```python
from build123d import *

# Parameters (mm, degrees)
SKETCH1_W           = 24
SKETCH1_H           = 9
BOSS_EXTRUDE1_DEPTH = 75
FILLET1_R           = 1
FILLET2_R           = 3
SKETCH2_R           = 2.5
CUT_EXTRUDE1_DEPTH  = 6
SKETCH3_R           = 2.5
CUT_EXTRUDE2_DEPTH  = 10
SKETCH4_R           = 5
CUT_EXTRUDE3_DEPTH  = 4


with BuildPart() as part:
    # Sketch1 → Boss-Extrude1 (new body)
    with BuildSketch(Plane.XY):
        Polygon((-18, -4.5), (-12, -4.5), (-12, 4.5), (-12, 14.5), (-18, 14.5), align=None)
        Rectangle(SKETCH1_W, SKETCH1_H)
        Polygon((12, 4.5), (12, -4.5), (18, -4.5), (18, 24.5), (12, 24.5), align=None)
    extrude(amount=BOSS_EXTRUDE1_DEPTH)

    # Fillet1
    fillet1_edges = [part.edges().sort_by_distance(p)[0] for p in [
        (-12, 4.5, 37.5),
        (12, 4.5, 37.5),
    ]]
    fillet(fillet1_edges, radius=FILLET1_R)

    # Fillet2
    fillet2_edges = [part.edges().sort_by_distance(p)[0] for p in [
        (18, 10, 0),
        (-18, 5, 0),
        (18, 10, 75),
        (-18, 5, 75),
    ]]
    fillet(fillet2_edges, radius=FILLET2_R)

    # Sketch2 → Cut-Extrude1 (cut)
    with BuildSketch(Plane.ZY.offset(-12)):
        with Locations((37.5, 13.5)):
            Circle(SKETCH2_R)
    extrude(amount=-CUT_EXTRUDE1_DEPTH, mode=Mode.SUBTRACT)

    # Sketch3 → Cut-Extrude2 (cut)
    with BuildSketch(Plane(origin=(0, 4.5, 0), x_dir=(1, 0, 0), z_dir=(0, 1, 0))):
        with Locations(Location((0, -37.5, 0), (0, 0, 270))):
            Circle(SKETCH3_R)
        with Locations(Location((0, -7.5, 0), (0, 0, 270))):
            Circle(SKETCH3_R)
        with Locations(Location((0, -67.5, 0), (0, 0, 270))):
            Circle(SKETCH3_R)
    extrude(amount=-CUT_EXTRUDE2_DEPTH, mode=Mode.SUBTRACT)

    # Sketch4 → Cut-Extrude3 (cut)
    with BuildSketch(Plane(origin=(0, 4.5, 0), x_dir=(1, 0, 0), z_dir=(0, 1, 0))):
        with Locations(Location((0, -7.5, 0), (0, 0, 270))):
            Circle(SKETCH4_R)
        with Locations(Location((0, -37.5, 0), (0, 0, 270))):
            Circle(SKETCH4_R)
        with Locations(Location((0, -67.5, 0), (0, 0, 270))):
            Circle(SKETCH4_R)
    extrude(amount=-CUT_EXTRUDE3_DEPTH, mode=Mode.SUBTRACT)


solid = part.part
```
Read the model definition and answer for the solid it produces. Units are mm, in the model's axes. A direction names the side the tool comes from. Coordinates: 2 decimals unless noted, no trailing zeros. Loops run counter-clockwise (first coordinate to the right, second up) from the corner with the lowest first, then second, coordinate; pieces in that order, holes last. Notation, with made-up numbers: (38.5, 19) - (70.5, 19) arc R21 cw to (70.5, 36) - close; hole circle Ø8 at (-36.75, 2). An arc over 180 degrees is marked (long way). Answer in a Markdown table with one row per item.
1. Straight lines are drawn through the part: line 1 (X direction, y = 7, z = 17); line 2 (X direction, y = 2.4, z = 67.5); line 3 (Z direction, x = 3, y = 2). For each, find the intervals that lie inside material, in ascending order.
Conclusion:
| item | result |
|---|---|
| line 1 | x = -18 to -12, 12 to 18 |
| line 2 | x = -18 to -5, 5 to 18 |
| line 3 | z = 0 to 3.5, 11.5 to 33.5, 41.5 to 63.5, 71.5 to 75 |
2. Find section A-A, the plane x = 0. Write down the section's boundary in (y, z), then the cut area to 3 significant figures.
Conclusion:
| item | result |
|---|---|
| outline | (-4.5, 0) - (4.5, 0) - (4.5, 2.5) - (0.5, 2.5) - (0.5, 5) - (-4.5, 5) - close; (-4.5, 10) - (0.5, 10) - (0.5, 12.5) - (4.5, 12.5) - (4.5, 32.5) - (0.5, 32.5) - (0.5, 35) - (-4.5, 35) - close; (-4.5, 40) - (0.5, 40) - (0.5, 42.5) - (4.5, 42.5) - (4.5, 62.5) - (0.5, 62.5) - (0.5, 65) - (-4.5, 65) - close; (-4.5, 70) - (0.5, 70) - (0.5, 72.5) - (4.5, 72.5) - (4.5, 75) - (-4.5, 75) - close |
| area | 480 mm² |
3. Given pin 1 (16 mm diameter, centred on x = 0, z = 7.5, fed in from -Y); pin 2 (8 mm diameter, centred on x = 0, z = 67.5, fed in from +Y); pin 3 (11 mm diameter, centred on x = -2.5, z = 32, fed in from +Y); pin 4 (5 mm diameter, centred on x = -15, z = 22, fed in from +Y), each flat-ended and moving along its own axis, determine where each tip first touches the part or whether it passes through.
Conclusion:
| item | result |
|---|---|
| pin 1 | stops at y = -4.5 |
| pin 2 | stops at y = 0.5 |
| pin 3 | stops at y = 4.5 |
| pin 4 | stops at y = 14.5 |
4. Find section B-B, the plane y = 10.25. Write down the section's boundary in (x, z), then the cut area to 3 significant figures.
Conclusion:
| item | result |
|---|---|
| outline | (-18, 3) arc R3 ccw to (-15, 0) - (-12, 0) - (-12, 75) - (-15, 75) arc R3 ccw to (-18, 72) - close; (12, 0) - (15, 0) arc R3 ccw to (18, 3) - (18, 72) arc R3 ccw to (15, 75) - (12, 75) - close |
| area | 892 mm² |
5. Which of the six approach directions +Z, -Z, +X, -X, +Y, -Y give full straight-line access (tool end or side, diameter ignored) to faces 1 (the face through (14.96, 12.54, 39.81)), 2 (the face through (-12, 10, 37)), 3 (the face through (1.5, 2.53, 12.27))?
Conclusion:
| item | result |
|---|---|
| face 1 | +X |
| face 2 | +Z, -Z, +Y |
| face 3 | +Y |
6. Find section D-D, the plane y = 13.5. Write down the section's boundary in (x, z), then the cut area to 3 significant figures.
Conclusion:
| item | result |
|---|---|
| outline | (-18, 3) arc R3 ccw to (-15, 0) - (-12, 0) - (-12, 75) - (-15, 75) arc R3 ccw to (-18, 72) - close; (12, 0) - (15, 0) arc R3 ccw to (18, 3) - (18, 35) - (12, 35) - close; (12, 40) - (18, 40) - (18, 72) arc R3 ccw to (15, 75) - (12, 75) - close |
| area | 862 mm² |
7. Determine the mould class of faces 4 (the face through (-17.1, 4.87, 0.86)), 5 (the face through (-1.915, 2.528, 72.119)), 6 (the face through (17.1, 10.2, 74.14)), 7 (the face through (-4, -4.5, 37)) for opening direction X: +X half, -X half, draft (parallel to the pull), parting line (faces both ways), or undercut.
Conclusion:
| item | result |
|---|---|
| face 4 | -X half |
| face 5 | undercut |
| face 6 | +X half |
| face 7 | draft |
8. Find section C-C, the plane z = 67.5. Write down the section's boundary in (x, y), then the cut area to 3 significant figures.
Conclusion:
| item | result |
|---|---|
| outline | (-18, -4.5) - (-2.5, -4.5) - (-2.5, 0.5) - (-5, 0.5) - (-5, 4.5) - (-11, 4.5) arc R1 cw to (-12, 5.5) - (-12, 14.5) - (-18, 14.5) - close; (2.5, -4.5) - (18, -4.5) - (18, 24.5) - (12, 24.5) - (12, 5.5) arc R1 cw to (11, 4.5) - (5, 4.5) - (5, 0.5) - (2.5, 0.5) - close |
| area | 439 mm² |
